Answer from the drawing. Dimensions are ordinates in mm from the lowest x, y and z of the part. Give positions to 0.01 mm unless a question says otherwise; leave off trailing zeros. Order: outer loops, then holes, each group sorted by start corner. A loop starts at its lowest first (then second) coordinate and runs counter-clockwise, first axis right, second up. Notation, with made-up numbers: (16.25, -9) -> (41.25, -9) arc R26 cw to (41.25, 24) -> close; hole circle Ø9 at (3, 82.25). An arc over 180 degrees is marked (long way). One line per question, with ' | ' between items. Start each with the question number.
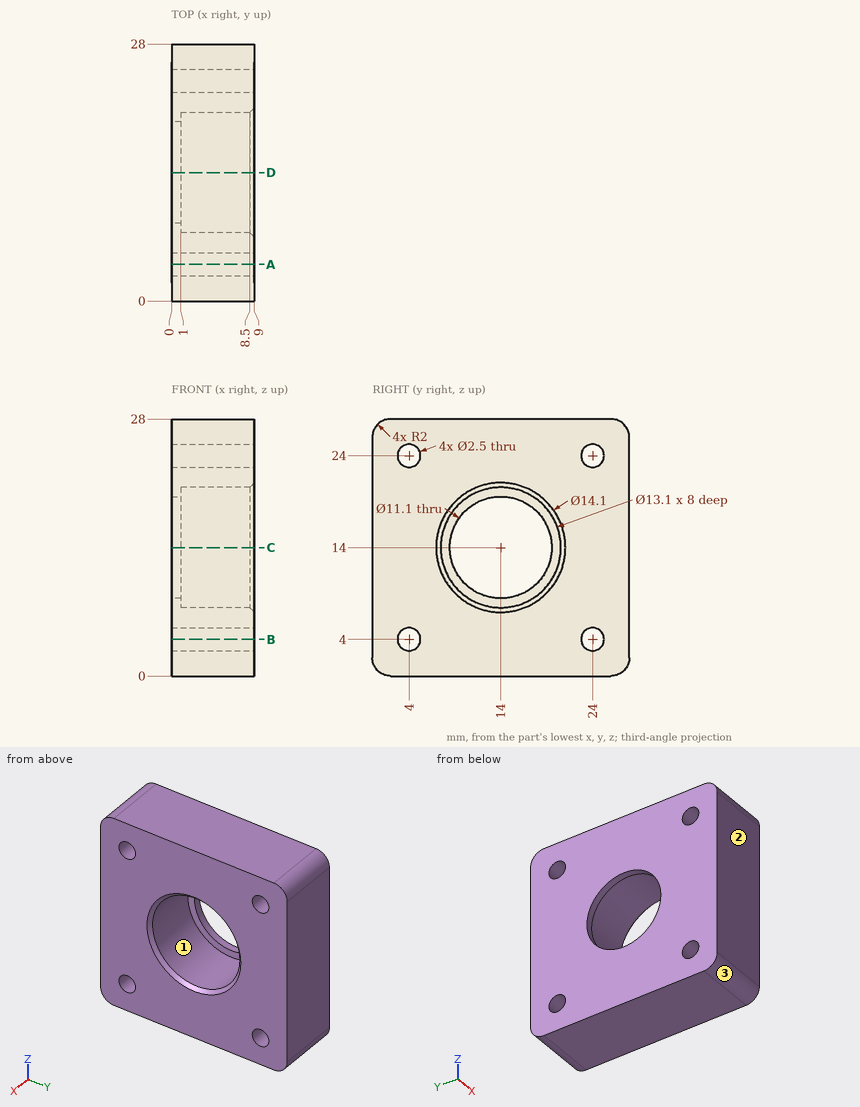
(1) The part is cut by section C-C on z = 14. Determine the outline of the cut face in (x, y), plus the area to 3 significant figures.
(2) Given P1, Ø2, axis at y = 24, z = 4, coming from the -X side; P2, Ø6.5, axis at y = 12, z = 12, coming from the +X side, each flat-ended and moving along its own axis, determine where each tip first touches the part or whether it passes through.
(3) The part is cut by section A-A on y = 4. Determine the outline of the cut face in (x, z).
(4) Consider line 1 (Y direction, x = 7, z = 4); line 2 (Y direction, x = 3.25, z = 13.75). Determine where each line is inside the solid, lowest interval first.
(5) Determine the mould class of the marked faces 1, 2 and 3 for opening direction Z: pulls with the +Z half, pulls with the -Z half, needs draft (parallel to the pull), parting line crosses it, or undercut.
Result sheet:
1) outline: (0, 0) -> (9, 0) -> (9, 6.95) -> (8.5, 7.45) -> (1, 7.45) -> (1, 8.45) -> (0, 8.45) -> close; (0, 19.55) -> (1, 19.55) -> (1, 20.55) -> (8.5, 20.55) -> (9, 21.05) -> (9, 28) -> (0, 28) -> close | area: 136 mm^2
2) P1: passes through | P2: stops at x = 1
3) outline: (0, 0) -> (9, 0) -> (9, 2.75) -> (0, 2.75) -> close; (0, 5.25) -> (9, 5.25) -> (9, 22.75) -> (0, 22.75) -> close; (0, 25.25) -> (9, 25.25) -> (9, 28) -> (0, 28) -> close
4) line 1: y = 0 to 2.75, 5.25 to 22.75, 25.25 to 28 | line 2: y = 0 to 7.45, 20.55 to 28
5) face 1: undercut | face 2: needs draft | face 3: pulls with the -Z half
